```python
from build123d import *

# Parameters (mm, degrees)
SKETCH1_W           = 126
SKETCH1_H           = 6
BOSS_EXTRUDE1_DEPTH = 4
SKETCH2_W           = 3
SKETCH2_H           = 3
CUT_EXTRUDE1_DEPTH  = 4
SKETCH3_W           = 10
SKETCH3_H           = 6
BOSS_EXTRUDE2_DEPTH = 20
SKETCH4_W           = 10
SKETCH4_H           = 4
BOSS_EXTRUDE3_DEPTH = 26
SKETCH5_W           = 6
SKETCH5_H           = 4
BOSS_EXTRUDE4_DEPTH = 42.5
SKETCH6_W           = 10
SKETCH6_H           = 4
BOSS_EXTRUDE5_DEPTH = 14


with BuildPart() as part:
    # Sketch1 → Boss-Extrude1 (new body)
    with BuildSketch(Plane(origin=(0, 0, 0), x_dir=(1, 0, 0), z_dir=(0, 1, 0))):
        with Locations((63, 3)):
            Rectangle(SKETCH1_W, SKETCH1_H)
    extrude(amount=BOSS_EXTRUDE1_DEPTH)

    # Sketch2 → Cut-Extrude1 (cut)
    with BuildSketch(Plane(origin=(0, 4, 0), x_dir=(1, 0, 0), z_dir=(0, 1, 0))):
        with Locations((121.5, 3)):
            Rectangle(SKETCH2_W, SKETCH2_H)
        with Locations((4.5, 3)):
            Rectangle(SKETCH2_W, SKETCH2_H)
    extrude(amount=-CUT_EXTRUDE1_DEPTH, mode=Mode.SUBTRACT)

    # Sketch3 → Boss-Extrude2 (add)
    with BuildSketch(Plane(origin=(0, 0, 0), x_dir=(1, 0, 0), z_dir=(0, 1, 0))):
        with Locations((14, 3)):
            Rectangle(SKETCH3_W, SKETCH3_H)
        with Locations((112, 3)):
            Rectangle(SKETCH3_W, SKETCH3_H)
        with Locations((37.5, 3)):
            Rectangle(SKETCH3_W, SKETCH3_H)
    extrude(amount=-BOSS_EXTRUDE2_DEPTH)

    # Sketch4 → Boss-Extrude3 (add)
    with BuildSketch(Plane(origin=(0, 0, -6), x_dir=(-1, 0, 0), z_dir=(0, 0, -1))):
        with Locations((-14, 2)):
            Rectangle(SKETCH4_W, SKETCH4_H)
        with Locations((-37.5, 2)):
            Rectangle(SKETCH4_W, SKETCH4_H)
    extrude(amount=BOSS_EXTRUDE3_DEPTH)

    # Sketch5 → Boss-Extrude4 (add)
    with BuildSketch(Plane(origin=(42.5, 0, 0), x_dir=(0, 0, -1), z_dir=(1, 0, 0))):
        with Locations((25, 2)):
            Rectangle(SKETCH5_W, SKETCH5_H)
        with Locations((3, -18)):
            Rectangle(SKETCH5_W, SKETCH5_H)
    extrude(amount=-BOSS_EXTRUDE4_DEPTH)

    # Sketch6 → Boss-Extrude5 (add)
    with BuildSketch(Plane(origin=(0, 0, -6), x_dir=(-1, 0, 0), z_dir=(0, 0, -1))):
        with Locations((-112, 2)):
            Rectangle(SKETCH6_W, SKETCH6_H)
    extrude(amount=BOSS_EXTRUDE5_DEPTH)


solid = part.part
```
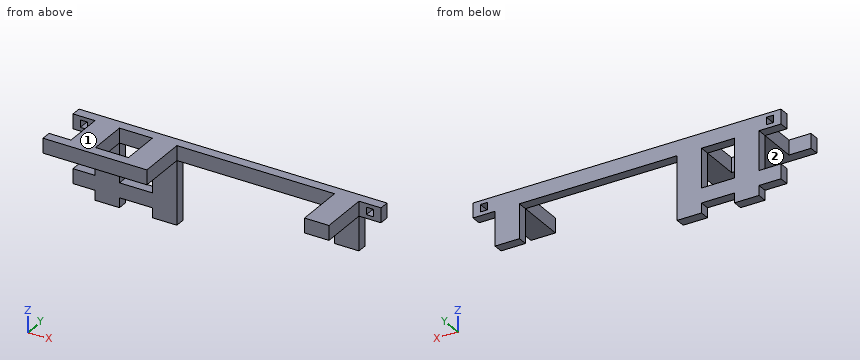
For this review, take the finished solid that the model builds, in its own axes (mm). Face numbers are marked on the shaded views. A direction names the side the tool comes from. Coordinates: 2 decimals unless noted, no trailing zeros. Write each loop counter-clockwise with the first axis right and the second up, starting at its lowest first coordinate (ties: lowest second). Pieces come first, ordered by that corner, then holes. Notation, with made-up numbers: (37.25, -21) - (82.25, -21) arc R12 cw to (82.25, -8) - close; hole circle Ø1 at (64.25, 71.25). An arc over 180 degrees is marked (long way). Answer in a Markdown table with one row per item. Add a question column.
Q1. We need section C-C, the plane z = -3. State the section outline as (x, y) points.
Q2. We need section D-D, the plane y = 1.75. Count the separate pieces of the cut face and the enclosed holes in it, and give its area (3 significant figures).
Q3. Tool access review of the marked faces 1 and 2: name each direction out of +Z, -Z, +X, -X, +Y, -Y from which nothing blocks a thin tool from reaching the whole face with its end or side.
Q4. We need section B-B, the plane x = 25. State the section outline as (y, z) points, and give its area (3 significant figures).
Q5. For probe 1 along X at (y, z) = (0.5, -10); probe 2 along Z at (x, y) = (112.5, -11.5); probe 3 along Y at (x, z) = (18, -26.5), list the stretches that pass through material, from the lowest coordinate up.
Q6. For P1, Ø1.2, axis at y = 2.5, z = -10, coming from the -X side; P2, Ø10, axis at x = 106, y = 1, coming from the -Z side; P3, Ø4, axis at x = 29.5, z = -18, coming from the -Y side; P4, Ø0.9, axis at x = 5, y = 3, coming from the -Z side, all flat-tipped, find the tip position at first contact; note any pin that passes through.
Q7. We need section A-A, the plane y = -8.5. State the section outline as (x, z) points, and give its area (3 significant figures).
Answer list:
| question | item | result |
|---|---|---|
| 1 | outline | (0, -20) - (42.5, -20) - (42.5, 0) - (107, 0) - (107, -20) - (117, -20) - (117, 0) - (120, 0) - (120, 4) - (6, 4) - (6, 0) - (9, 0) - (9, -16) - (0, -16) - close; (0, 0) - (3, 0) - (3, 4) - (0, 4) - close; (123, 0) - (126, 0) - (126, 4) - (123, 4) - close; hole (19, -16) - (32.5, -16) - (32.5, 0) - (19, 0) - close |
| 2 | separate pieces | 1 |
| 2 | enclosed holes | 3 |
| 2 | area | 1,530 mm2 |
| 3 | face 1 | +Z, +X, -X, +Y, -Y |
| 3 | face 2 | -Z, +X, -X, -Y |
| 4 | outline | (-20, -6) - (-16, -6) - (-16, 0) - (-20, 0) - close; (0, -28) - (4, -28) - (4, -22) - (0, -22) - close; (0, -6) - (4, -6) - (4, 0) - (0, 0) - close |
| 4 | area | 72.0 mm2 |
| 5 | probe 1 | x = 9 to 19, 32.5 to 42.5, 107 to 117 |
| 5 | probe 2 | z = -6 to 0 |
| 5 | probe 3 | y = 0 to 4 |
| 6 | P1 | stops at x = 9 |
| 6 | P2 | stops at z = -20 |
| 6 | P3 | passes through |
| 6 | P4 | stops at z = -28 |
| 7 | outline | (9, -6) - (19, -6) - (19, 0) - (9, 0) - close; (32.5, -6) - (42.5, -6) - (42.5, 0) - (32.5, 0) - close; (107, -6) - (117, -6) - (117, 0) - (107, 0) - close |
| 7 | area | 180 mm2 |
